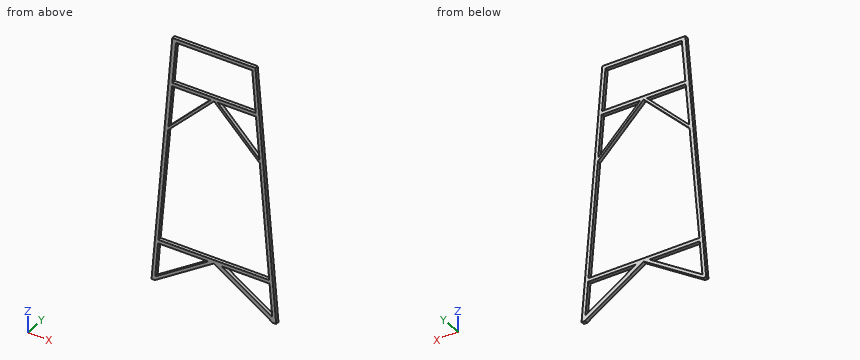
```python
from build123d import *

# Parameters (mm, degrees)
F1_DEPTH = 25.4


# Not quite as in the source:
# - a feature names something its author has since deleted; it is built from what else it names


with BuildPart() as f1:
    # F0 (on Front) → F1 (new body)
    with BuildSketch(Plane.XZ):
        Polygon((0, 358.2734752655), (-304.8, 358.2734752655), (-457.2, -1470.5265247345), (-431.8, -1470.5265247337), (-0.1234569215, -1191.2064086248), (-1e-10, -1191.1265247345), (0.1234569213, -1191.2064086248), (431.8, -1470.5265247345), (457.2, -1470.5265247345), (304.8, 358.2734752655), align=None)
        Polygon((-429.5392940648, -1442.1890979106), (-409.5163731819, -1191.2064086248), (-41.6569560767, -1191.2064086248), align=None, mode=Mode.SUBTRACT)
        Polygon((0, -1165.7265247345), (-407.2488822076, -1164.9444627713), (-335.1759464959, -330.2), (1.7004121065, 2.7614467587), (336.7727896055, -330.2), (406.4, -1165.7265247345), align=None, mode=Mode.SUBTRACT)
        Polygon((57.3942214249, -1191.2064086248), (408.5233236575, -1191.2064086248), (428.535863163, -1431.3568826906), align=None, mode=Mode.SUBTRACT)
        Polygon((-23.6995878935, 2.7614467587), (-332.9828770612, -304.8), (-306.4276168969, 2.7614467587), align=None, mode=Mode.SUBTRACT)
        Polygon((334.6561229388, -304.8), (27.1003926271, 2.7299896004), (309.0577234879, 2.380793411), align=None, mode=Mode.SUBTRACT)
        Polygon((-277.9249521719, 332.8776175298), (281.5093551883, 332.9612130061), (306.9093551883, 28.1612130061), (-304.2345555955, 28.1613525589), align=None, mode=Mode.SUBTRACT)
    extrude(amount=F1_DEPTH)


solid = f1.part
```
CAD build for the part. Positions are in the model's coordinates, mm. Coordinates: 2 decimals unless noted, no trailing zeros. Order: outer loops, then holes, each group sorted by start corner. A loop starts at its lowest first (then second) coordinate and runs counter-clockwise, first axis right, second up. Notation, with made-up numbers: (24, 22) -> (62, 22) arc R22 ccw to (62, 34) -> close; hole circle Ø11 at (30.5, 63.5). An arc over 180 degrees is marked (long way). Use one line per item in the form item = value. Start each with the question number.
1) Band-saw the part on C-C on z = -217.5. Give the cut face in (x, y), then the cut area to 3 significant figures.
2) Drill centre lines: L1, parallel to X at y = -17.75, z = -199.5; L2, parallel to Z at x = -276, y = -8.5; L3, parallel to X at y = -13, z = -163.5. Where is each one in solid material? Low to high. Write a range as [from, to].
3) Drop flat-ended pins along their axis: pin 1 (7.5 mm diameter, centred on x = -188.5, y = -7.5, fed in from -Z); pin 2 (12.5 mm diameter, centred on x = -209.5, y = -9.5, fed in from -Z); pin 3 (12 mm diameter, centred on y = -6.5, z = -563.5, fed in from +X). Give the stop position or say it passes through.
4) Band-saw the part on D-D on z = -669. Give the cut face in (x, y), then the cut area to 3 significant figures.
5) Band-saw the part on B-B on x = -159. Give the cut face in (y, z), then the cut area to 3 significant figures.
6) Band-saw the part on A-A on y = -12.75. State how many separate pieces and enclosed holes the cut face has, then the cut area to 3 significant figures.
Entries:
q1.outline = (-352.78, -25.4) -> (-325.45, -25.4) -> (-325.45, 0) -> (-352.78, 0) -> close; (-245.19, -25.4) -> (-221.15, -25.4) -> (-221.15, 0) -> (-245.19, 0) -> close; (223.36, -25.4) -> (247.35, -25.4) -> (247.35, 0) -> (223.36, 0) -> close; (327.38, -25.4) -> (352.78, -25.4) -> (352.78, 0) -> (327.38, 0) -> close
q1.area = 2,560 mm2
q2.L1 = [-351.28, -323.89], [-227.09, -202.94], [205.24, 229.35], [325.88, 351.28]
q2.L2 = [-1369.71, -1342.84], [-1191.21, -1165.2], [-271.71, -248.13], [2.76, 28.16], [332.88, 358.27]
q2.L3 = [-348.28, -320.78], [-190.89, -166.52], [169.02, 193.34], [322.88, 348.28]
q3.pin_1 = -1315.52
q3.pin_2 = -1330.73
q3.pin_3 = 382.11
q4.outline = (-390.41, -25.4) -> (-364.43, -25.4) -> (-364.43, 0) -> (-390.41, 0) -> close; (365.01, -25.4) -> (390.41, -25.4) -> (390.41, 0) -> (365.01, 0) -> close
q4.area = 1,300 mm2
q5.outline = (-25.4, -1294.01) -> (0, -1294.01) -> (0, -1267.13) -> (-25.4, -1267.13) -> close; (-25.4, -1191.21) -> (0, -1191.21) -> (0, -1165.42) -> (-25.4, -1165.42) -> close; (-25.4, -156.07) -> (0, -156.07) -> (0, -131.79) -> (-25.4, -131.79) -> close; (-25.4, 2.76) -> (0, 2.76) -> (0, 28.16) -> (-25.4, 28.16) -> close; (-25.4, 332.9) -> (0, 332.9) -> (0, 358.27) -> (-25.4, 358.27) -> close
q5.area = 3,240 mm2
q6.separate_pieces = 1
q6.enclosed_holes = 6
q6.area = 187,000 mm2
